The model under review builds one solid part; all positions refer to its coordinate system, in mm. A direction names the side the tool comes from. Coordinates: 2 decimals unless noted, no trailing zeros. Order: outer loops, then holes, each group sorted by start corner. A loop starts at its lowest first (then second) coordinate and runs counter-clockwise, first axis right, second up. Notation, with made-up numbers: (53, 77) -> (91, 77) arc R29 ccw to (91, 104) -> close; hole circle Ø9 at (-21, 54.5). An arc over 180 degrees is marked (long way). Use CSV: the item, a comma, the result in double quotes. Start each with the question number.
```python
from build123d import *

# Parameters (mm, degrees)
SKETCH_R         = 6.095
SKETCH_R_2       = 4.8895
PAD_DEPTH        = 215
HOLE_D           = 3.05
HOLE_DEPTH       = 25
HOLE_CBORE_D     = 7.62
HOLE_CBORE_DEPTH = 5
SKETCH002_R      = 1.525
HOLE001_DEPTH    = 25


with BuildPart() as part:
    # Sketch → Pad (new body)
    with BuildSketch(Plane.XZ):
        Circle(SKETCH_R)
        Circle(SKETCH_R_2, mode=Mode.SUBTRACT)
    extrude(amount=PAD_DEPTH)

    # Hole
    with Locations(Plane.XY.offset(7)):
        with Locations((0, -207.79)):
            CounterBoreHole(HOLE_D / 2, HOLE_CBORE_D / 2, HOLE_CBORE_DEPTH, depth=HOLE_DEPTH)

    # Sketch002 → Hole001 (cut)
    with BuildSketch(Plane.XY.offset(7)):
        with Locations((0, -5)):
            Circle(SKETCH002_R)
        with Locations((0, -90)):
            Circle(SKETCH002_R)
    extrude(amount=-HOLE001_DEPTH, mode=Mode.SUBTRACT)


solid = part.part
```
Q1. Clearance check with flat-ended pins moving along their axes: pin 1 Ø2 at (y, z) = (-94, -0.5) entering from +X (3 decimals); pin 2 Ø1.5 at (x, y) = (-3, -130) entering from -Z; pin 3 Ø1.8 at (x, y) = (0, -90) entering from +Z; pin 4 Ø2 at (y, z) = (-27, -3) entering from -X. State where each tip first meets the part, or that it passes through.
Q2. Draft analysis for pull direction X (two halves, no side actions). For faces 1 (the cylindrical face through (-1.06, -105.995, -4.773)), 2 (the cylindrical face through (3.277, -105.995, 5.139)), 3 (the flat face through (-5, -215, 2)), state which applies: +X half, -X half, draft (parallel to the pull), parting line (faces both ways), or undercut.
Q3. Add section A-A, the plane z = 0. State the section outline as (x, y) points (1 decimal), then the cut area to 3 significant figures.
Q4. For faces 4 (the flat face through (-5, 0, 2)), 5 (the cylindrical face through (-3.02, -210.11, 4.61)), list the 3-axis set-ups (+Z, -Z, +X, -X, +Y, -Y) from which the entire face can be reached by the end or side of a thin tool; tool diameter is ignored.
Q5. To check wall thickness, follow probe 1 along Y at (x, z) = (0, -5.75) (3 decimals); probe 2 along Y at (x, z) = (0, 5.2) (3 decimals); probe 3 along Z at (x, y) = (-0.5, -125). State the ranges of each line that lie inside material, in increasing order.
Q6. Add section B-B, the plane y = -124. State the section outline as (x, z) points (1 decimal).
Answer block:
1,pin 1,"stops at x = 6.095"
1,pin 2,"stops at z = -5.66"
1,pin 3,"passes through"
1,pin 4,"stops at x = -5.76"
2,face 1,"undercut"
2,face 2,"parting line"
2,face 3,"draft"
3,outline,"(-6.1, -215) -> (-4.9, -215) -> (-4.9, 0) -> (-6.1, 0) -> close; (4.9, -215) -> (6.1, -215) -> (6.1, 0) -> (4.9, 0) -> close"
3,area,"518 mm²"
4,face 4,"+Z, -Z, +X, -X, +Y"
4,face 5,"+Z"
5,probe 1,"y = -215 to -209.315, -206.265 to -91.525, -88.475 to -6.525, -3.475 to 0"
5,probe 2,"y = -215 to -211.6, -203.98 to -91.525, -88.475 to -6.525, -3.475 to 0"
5,probe 3,"z = -6.07 to -4.86, 4.86 to 6.07"
6,outline,"circle Ø12.2 at (0, 0); hole circle Ø9.8 at (0, 0)"
